Job drawing, mm, ordinate dimensions from the low corner. One solid piece. A direction names the side the tool comes from. Give positions to 0.01 mm unless a question says otherwise; leave off trailing zeros. Write each loop counter-clockwise with the first axis right and the second up, starting at its lowest first coordinate (ties: lowest second). Pieces come first, ordered by that corner, then holes. Notation, with made-up numbers: (16, 48) - (75, 48) arc R19 cw to (75, 84) - close; hole circle Ø6 at (81.25, 89). An arc over 180 degrees is marked (long way). Answer in a Markdown table with one row per item. Add a question column.
1. Probe line 1 along X through (y, z) = (5, 2.25); line 2 along Y through (x, z) = (6.88, 4.25); line 3 along Z through (x, y) = (7, 8.5). List the from-to ranges inside material, lowest first.
2. Band-saw the part on B-B on x = 6.88. Write the cut outline in (y, z).
3. Band-saw the part on D-D on y = 2.25. Write the cut outline in (x, z), plus the area to 3 significant figures.
4. Drop a flat-ended pin along its axis: pin 1 Ø5 at (x, y) = (8.5, 3) entering from +Z. Give the stop position or say it passes through.
5. Pull direction Y, two halves, no side cores. Call the marked faces 1, 2 and 3: released by +Y, released by -Y, zero draft, split by the parting line, or undercut.
6. Band-saw the part on C-C on z = 3.5. Write the cut outline in (x, y).
7. Which spindle directions (+Z, -Z, +X, -X, +Y, -Y) get a long thin tool onto all of the face, cutting with end or side? Do the marked faces 4 and 5. Say none if no direction does.
8. Band-saw the part on A-A on y = 5.08. Write the cut outline in (x, z), plus the area to 3 significant figures.
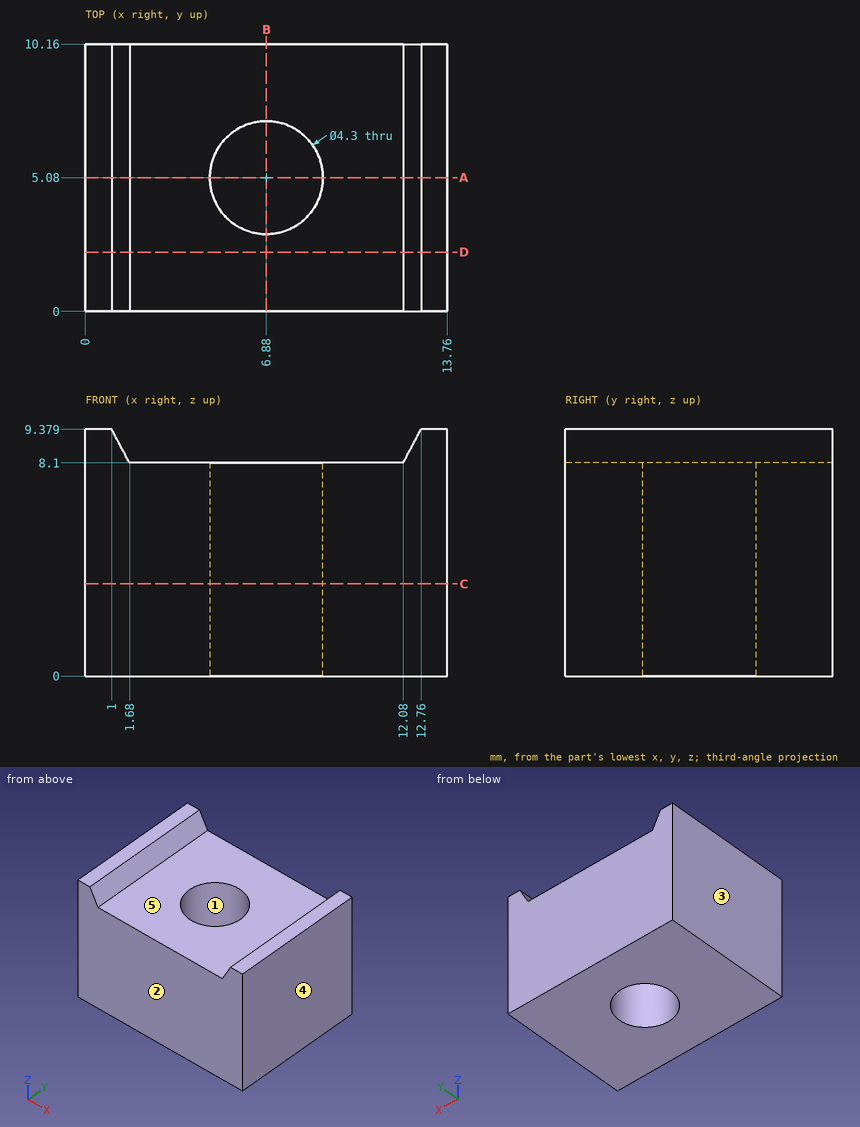
Values:
| question | item | result |
|---|---|---|
| 1 | line 1 | x = 0 to 4.73, 9.03 to 13.76 |
| 1 | line 2 | y = 0 to 2.93, 7.23 to 10.16 |
| 1 | line 3 | z = 0 to 8.1 |
| 2 | outline | (0, 0) - (2.93, 0) - (2.93, 8.1) - (0, 8.1) - close; (7.23, 0) - (10.16, 0) - (10.16, 8.1) - (7.23, 8.1) - close |
| 3 | outline | (0, 0) - (13.76, 0) - (13.76, 9.38) - (12.76, 9.38) - (12.08, 8.1) - (1.68, 8.1) - (1, 9.38) - (0, 9.38) - close |
| 3 | area | 115 mm² |
| 4 | pin 1 | stops at z = 8.1 |
| 5 | face 1 | undercut |
| 5 | face 2 | released by -Y |
| 5 | face 3 | zero draft |
| 6 | outline | (0, 0) - (13.76, 0) - (13.76, 10.16) - (0, 10.16) - close; hole circle Ø4.3 at (6.88, 5.08) |
| 7 | face 4 | +Z, -Z, +X, +Y, -Y |
| 7 | face 5 | +Z, +Y, -Y |
| 8 | outline | (0, 0) - (4.73, 0) - (4.73, 8.1) - (1.68, 8.1) - (1, 9.38) - (0, 9.38) - close; (9.03, 0) - (13.76, 0) - (13.76, 9.38) - (12.76, 9.38) - (12.08, 8.1) - (9.03, 8.1) - close |
| 8 | area | 80.1 mm² |
